```python
from build123d import *

# Parameters (mm, degrees)
F1_DEPTH  = 25.4
F2_R      = 6.35
F3_DEPTH  = 57.15
F5_DEPTH  = 31.75
F7_DEPTH  = 19.05
F9_DEPTH  = 12.7
F11_DEPTH = 12.7


with BuildPart() as f1:
    # F0 (on Front) → F1 (new body)
    with BuildSketch(Plane.XZ):
        Polygon((-36.3545019062, 31.75), (-61.7545019062, 31.75), (-61.7545019062, 0), (14.4454980938, 0), (14.4454980938, 12.7), (-36.3545019062, 12.7), align=None)
    extrude(amount=F1_DEPTH)

    # F2 (on face) → F3 (cut)
    with BuildSketch(Plane.XY.offset(31.75)):
        with Locations((-49.0545019062, -12.7)):
            Circle(F2_R)
    extrude(amount=-F3_DEPTH, mode=Mode.SUBTRACT)

    # F4 (on face) → F5 (cut)
    with BuildSketch(Plane.XY.offset(31.75)):
        with BuildLine():
            ThreePointArc((-61.7545019062, -12.6999997152), (-58.0347579265, -3.7197437782), (-49.0545019062, 0))
            Line((-49.0545019062, 0), (-61.7545019062, 0))
            Line((-61.7545019062, 0), (-61.7545019062, -12.6999997152))
        make_face()
        with BuildLine():
            Line((-61.7545019062, -25.4), (-49.0545019062, -25.4))
            ThreePointArc((-49.0545019062, -25.4), (-58.0347581279, -21.6802560204), (-61.7545019062, -12.6999997152))
            Line((-61.7545019062, -12.6999997152), (-61.7545019062, -25.4))
        make_face()
    extrude(amount=-F5_DEPTH, mode=Mode.SUBTRACT)

    # F6 (on face) → F7 (cut)
    with BuildSketch(Plane.XY.offset(31.75)):
        with BuildLine():
            ThreePointArc((-49.0545019062, 0), (-40.0742457851, -3.7197438789), (-36.3545019062, -12.7))
            Line((-36.3545019062, -12.7), (-36.3545019062, 0))
            Line((-36.3545019062, 0), (-49.0545019062, 0))
        make_face()
        with BuildLine():
            Line((-36.3545019062, -25.4), (-36.3545019062, -12.7))
            ThreePointArc((-36.3545019062, -12.7), (-40.0742457851, -21.6802561211), (-49.0545019062, -25.4))
            Line((-49.0545019062, -25.4), (-36.3545019062, -25.4))
        make_face()
    extrude(amount=-F7_DEPTH, mode=Mode.SUBTRACT)

    # F8 (on face) → F9 (cut)
    with BuildSketch(Plane.XY.offset(12.7)):
        with BuildLine():
            ThreePointArc((-23.6545019062, -19.05), (-19.1643738456, -17.1901280605), (-17.3045019062, -12.7))
            ThreePointArc((-17.3045019062, -12.7), (-19.1643738456, -8.2098719395), (-23.6545019062, -6.35))
            ThreePointArc((-23.6545019062, -6.35), (-30.0045019062, -12.7), (-23.6545019062, -19.05))
        make_face()
        with BuildLine():
            ThreePointArc((-23.6545019062, -6.35), (-19.1643738456, -8.2098719395), (-17.3045019062, -12.7))
            ThreePointArc((-17.3045019062, -12.7), (-19.1643738456, -17.1901280605), (-23.6545019062, -19.05))
            Line((-23.6545019062, -19.05), (1.7454980938, -19.05))
            ThreePointArc((1.7454980938, -19.05), (-4.6045019062, -12.7), (1.7454980938, -6.35))
            Line((1.7454980938, -6.35), (-23.6545019062, -6.35))
        make_face()
        with BuildLine():
            ThreePointArc((8.0954980938, -12.7), (6.2356261544, -8.2098719395), (1.7454980938, -6.35))
            ThreePointArc((1.7454980938, -6.35), (-4.6045019062, -12.7), (1.7454980938, -19.05))
            ThreePointArc((1.7454980938, -19.05), (6.2356261544, -17.1901280605), (8.0954980938, -12.7))
        make_face()
    extrude(amount=-F9_DEPTH, mode=Mode.SUBTRACT)

    # F10 (on face) → F11 (cut)
    with BuildSketch(Plane.XY.offset(12.7)):
        with BuildLine():
            ThreePointArc((1.7454980938, 0), (10.7257542149, -3.7197438789), (14.4454980938, -12.7))
            Line((14.4454980938, -12.7), (14.4454980938, 0))
            Line((14.4454980938, 0), (1.7454980938, 0))
        make_face()
        with BuildLine():
            Line((14.4454980938, -25.4), (14.4454980938, -12.7))
            ThreePointArc((14.4454980938, -12.7), (10.7257542149, -21.6802561211), (1.7454980938, -25.4))
            Line((1.7454980938, -25.4), (14.4454980938, -25.4))
        make_face()
    extrude(amount=-F11_DEPTH, mode=Mode.SUBTRACT)


solid = f1.part
```
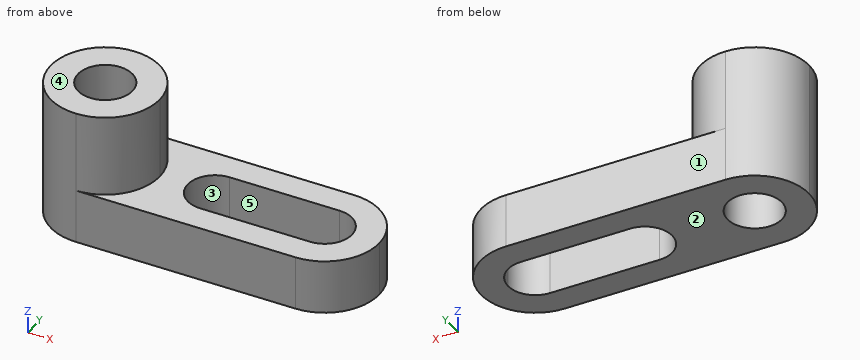
CAD build for the part. Positions are in the model's coordinates, mm. Face numbers are marked on the shaded views. A direction names the side the tool comes from. Round coordinates to 2 decimals unless told otherwise and drop trailing zeros. Order: outer loops, then holes, each group sorted by start corner. A loop starts at its lowest first (then second) coordinate and runs counter-clockwise, first axis right, second up.
Q1. Slice it at C-C (z = 4.5). Write the cut outline in (x, y).
Q2. Slice it at A-A (x = -22). Write the cut outline in (y, z).
Q3. Slice it at D-D (x = -38). Write the cut outline in (y, z), and give its area (3 significant figures).
Q4. Wall check: L1, parallel to Y at x = -0.5, z = 8; L2, parallel to X at y = -16.75, z = 3.5; L3, parallel to X at y = -13.5, z = 2.5. Give the ranges that are in metal, low to high.
Q5. Two-plate mould, pull along Y, no slides. Class the marked faces 1, 2 and 3: pulls with the +Y half, pulls with the -Y half, needs draft (parallel to the pull), parting line crosses it, or undercut.
Q6. Which spindle directions (+Z, -Z, +X, -X, +Y, -Y) get a long thin tool onto all of the face, cutting with end or side? Do the marked faces 4 and 5. Say none if no direction does.
Q7. Slice it at B-B (y = -16.75). Write the cut outline in (x, z), and give its area (3 significant figures).
Q8. Drop flat-ended pins along their axis: pin 1 (2 mm diameter, centred on y = -22, z = 8, fed in from +X); pin 2 (6 mm diameter, centred on x = -19.5, y = -18.5, fed in from +Z); pin 3 (5 mm diameter, centred on y = -8.5, z = 16.5, fed in from +X); pin 4 (4 mm diameter, centred on x = -5.5, y = -8.5, fed in from -Z). Give the stop position or say it passes through.
Results below:
1. outline: (-49.05, -25.4) - (1.75, -25.4) arc R12.7 ccw to (1.75, 0) - (-49.05, 0) arc R12.7 ccw to start; hole circle Ø12.7 at (-49.05, -12.7); hole (-23.65, -19.05) - (1.75, -19.05) arc R6.35 ccw to (1.75, -6.35) - (-23.65, -6.35) arc R6.35 ccw to start
2. outline: (-25.4, 0) - (-19.05, 0) - (-19.05, 12.7) - (-25.4, 12.7) - close; (-6.35, 0) - (0, 0) - (0, 12.7) - (-6.35, 12.7) - close
3. outline: (-25.4, 0) - (0, 0) - (0, 12.7) - (-6.45, 12.7) - (-6.45, 31.75) - (-18.95, 31.75) - (-18.95, 12.7) - (-25.4, 12.7) - close
3. area: 561 mm2
4. L1: y = -25.4 to -19.05, -6.35 to 0
4. L2: x = -61.09 to -53.95, -44.16 to -28.55, 6.64 to 13.78
4. L3: x = -61.73 to -55.35, -42.76 to -29.95, 8.04 to 14.42
5. face 1: pulls with the +Y half
5. face 2: needs draft
5. face 3: undercut
6. face 4: +Z, +X, -X, +Y, -Y
6. face 5: +Z, -Z
7. outline: (-61.09, 0) - (-53.95, 0) - (-53.95, 31.75) - (-61.09, 31.75) - close; (-44.16, 0) - (-28.55, 0) - (-28.55, 12.7) - (-37.02, 12.7) - (-37.02, 31.75) - (-44.16, 31.75) - close; (6.64, 0) - (13.78, 0) - (13.78, 12.7) - (6.64, 12.7) - close
7. area: 652 mm2
8. pin 1: stops at x = 11.36
8. pin 2: stops at z = 12.7
8. pin 3: stops at x = -36.47
8. pin 4: passes through
